from build123d import *

# Parameters (mm, degrees)
BOSS_EXTRUDE1_DEPTH = 6.25
CUT_EXTRUDE1_DEPTH  = 10
BOSS_EXTRUDE2_DEPTH = 6.25
CUT_EXTRUDE2_START  = -1.5
CUT_EXTRUDE2_DEPTH  = 1.5
MOVE_FACE1_BY       = 0.25
SKETCH5_R           = 1.3
CUT_EXTRUDE3_DEPTH  = 0.4
BOSS_EXTRUDE3_DEPTH = 6.25
MOVE_FACE2_BY       = 0.5
MOVE_FACE2_2_BY     = 0.5
CUT_EXTRUDE4_DEPTH  = 13
CUT_EXTRUDE5_START  = -1.5
CUT_EXTRUDE5_DEPTH  = 1.5
BOSS_EXTRUDE4_DEPTH = 6.25
CUT_EXTRUDE6_DEPTH  = 9.000000000000002
FILLET1_R           = 1
FILLET2_R           = 0.3


with BuildPart() as part:
    # Sketch1 → Boss-Extrude1 (new body)
    with BuildSketch(Plane(origin=(0, 0, 0), x_dir=(1, 0, 0), z_dir=(0, 1, 0))):
        with BuildLine():
            Line((-8.500000000000007, 21.49999999999999), (-8.500000000000007, 15.499999999999982))
            Line((-8.500000000000007, 15.499999999999982), (16.645822822062563, 5.999999999999995))
            Line((16.645822822062563, 5.999999999999995), (20.645822822062566, 5.999999999999995))
            ThreePointArc((20.645822822062566, 5.999999999999995), (12.90833064342558, 17.19374886404939), (0, 21.49999999999999))
            Line((0, 21.49999999999999), (-8.500000000000007, 21.49999999999999))
        make_face()
    extrude(amount=BOSS_EXTRUDE1_DEPTH)

    # Sketch2 → Cut-Extrude1 (cut)
    with BuildSketch(Plane(origin=(0, 6.25, 0), x_dir=(1, 0, 0), z_dir=(0, 1, 0))):
        with BuildLine():
            Line((-9.752670250943163, 2.7674418604651105), (-9.752670250943163, 14.499999999999986))
            Line((-9.752670250943163, 14.499999999999986), (8.3e-16, 14.499999999999986))
            ThreePointArc((8.3e-16, 14.499999999999986), (9.22285457500159, 11.188786953390961), (14.233455854041384, 2.7674418604651105))
            Line((14.233455854041384, 2.7674418604651105), (-9.752670250943163, 2.7674418604651105))
        make_face()
    extrude(amount=-CUT_EXTRUDE1_DEPTH, mode=Mode.SUBTRACT)

    # Sketch3 → Boss-Extrude2 (add)
    with BuildSketch(Plane(origin=(0, 6.25, 0), x_dir=(1, 0, 0), z_dir=(0, 1, 0))):
        Polygon((4.469156931645221, 10.801748174518188), (6.3032770804154685, 10.004250036667695), (8.404211615552752, 14.836068669534448), (2.8125557708062745, 17.02319772649103), (0.8009166341047183, 12.396744450219176), (2.6350367828749666, 11.599246312368683), align=None)
    extrude(amount=-BOSS_EXTRUDE2_DEPTH)

    # Sketch4 → Cut-Extrude2 (cut)
    with BuildSketch(Plane.XZ.offset(CUT_EXTRUDE2_START)):
        with BuildLine():
            Line((12.329816757236909, -7.63057132415126), (4.858273185949837, -3.0066464723283906))
            Line((4.858273185949837, -3.0066464723283906), (-2.1755255087838874, -6.757515163827213))
            Line((-2.1755255087838874, -6.757515163827213), (0.39188162426461154, -14.49470347377149))
            ThreePointArc((0.39188162426461154, -14.49470347377149), (7.227688425031692, -12.570223547362334), (12.329816757236909, -7.63057132415126))
        make_face()
    extrude(amount=CUT_EXTRUDE2_DEPTH, mode=Mode.SUBTRACT)

    # Move Face1: a face moved outward by 0.25
    extrude(part.faces().sort_by_distance((3.552096857, 3.875, -11.200497243))[0], amount=MOVE_FACE1_BY, dir=(-0.398749069, 0, 0.917060074))

    # Sketch5 → Cut-Extrude3 (cut)
    with BuildSketch(Plane(origin=(4.560861605165302, 0, -10.489263571615414), x_dir=(0.917060074385124, 0, 0.3987490689252462), z_dir=(-0.3987490689252462, 0, 0.917060074385124))):
        with Locations((-1.20870163918075, 3.2500000000000084)):
            Circle(SKETCH5_R)
    extrude(amount=-CUT_EXTRUDE3_DEPTH, mode=Mode.SUBTRACT)

    # Sketch6 → Boss-Extrude3 (add)
    with BuildSketch(Plane(origin=(0, 6.25, 0), x_dir=(1, 0, 0), z_dir=(0, 1, 0))):
        Polygon((-8.500000000000007, 15.900685410943252), (-8.398385997633637, 15.900685410943252), (-8.398385997633637, 17.900685410943254), (-8.500000000000007, 17.900685410943254), (-10.500000000000009, 17.900685410943254), (-10.500000000000009, 15.900685410943252), align=None)
    extrude(amount=-BOSS_EXTRUDE3_DEPTH)

    # Move Face2: a face moved inward by 0.5
    extrude(part.faces().sort_by_distance((-4.25, 3.125, -21.5))[0], amount=MOVE_FACE2_BY, dir=(0, 0, 1), mode=Mode.SUBTRACT)

    # Move Face2 2: a curved face moved inward by 0.5
    add(Solid.thicken(part.faces().sort_by_distance((12.908330643, 3.125, -17.193748864))[0], -MOVE_FACE2_2_BY), mode=Mode.SUBTRACT)

    # Sketch7 → Cut-Extrude4 (cut)
    with BuildSketch(Plane(origin=(0, 6.25, 0), x_dir=(1, 0, 0), z_dir=(0, 1, 0))):
        with BuildLine():
            Line((-8.500000000000007, 15.900685410943252), (0, 15.900685410943252))
            ThreePointArc((0, 15.900685410943252), (1.1301672935759872, 15.860470309114884), (2.2546178785171396, 15.740028423089157))
            Line((2.2546178785171396, 15.740028423089157), (1.4365096738849472, 13.858508365832973))
            Line((1.4365096738849472, 13.858508365832973), (0.7012293668734065, 12.167479431622894))
            Line((0.7012293668734065, 12.167479431622894), (6.203589813184157, 9.774985018071414))
            Line((6.203589813184157, 9.774985018071414), (7.238188726101288, 12.15439961732261))
            Line((7.238188726101288, 12.15439961732261), (7.94274956604829, 13.774778614149243))
            ThreePointArc((7.94274956604829, 13.774778614149243), (13.653169200208351, 8.150016400490594), (15.89419526397822, 0.45426143168428607))
            Line((15.89419526397822, 0.45426143168428607), (-20.808588691152597, -0.594716444159659))
            Line((-20.808588691152597, -0.594716444159659), (-15.374732718008488, 14.86339738490728))
            Line((-15.374732718008488, 14.86339738490728), (-8.500000000000007, 15.900685410943252))
        make_face()
    extrude(amount=-CUT_EXTRUDE4_DEPTH, mode=Mode.SUBTRACT)

    # Sketch8 → Cut-Extrude5 (cut)
    with BuildSketch(Plane.XZ.offset(CUT_EXTRUDE5_START)):
        with BuildLine():
            Line((14.339308110473954, -6.871392831928589), (1.9043764034639075, -3.0604478341676384))
            Line((1.9043764034639075, -3.0604478341676384), (-4.2629376925202305, -10.324173324993405))
            Line((-4.2629376925202305, -10.324173324993405), (0.7554626751993575, -15.882728754347104))
            ThreePointArc((0.7554626751993575, -15.882728754347104), (8.789998296056245, -13.250197224687337), (14.339308110473954, -6.871392831928589))
        make_face()
    extrude(amount=CUT_EXTRUDE5_DEPTH, mode=Mode.SUBTRACT)

    # Sketch9 → Boss-Extrude4 (add)
    with BuildSketch(Plane(origin=(0, 6.25, 0), x_dir=(1, 0, 0), z_dir=(0, 1, 0))):
        with BuildLine():
            Line((15.70292318448331, 2.500000000000002), (17.725251454235494, 2.500000000000002))
            ThreePointArc((17.725251454235494, 2.500000000000002), (16.78932753436898, 6.209107831207082), (15.086677514257817, 9.634661420966763))
            Line((15.086677514257817, 9.634661420966763), (13.225064123719731, 8.827767297640147))
            ThreePointArc((13.225064123719731, 8.827767297640147), (14.805987713393527, 5.797803408931993), (15.70292318448331, 2.500000000000002))
        make_face()
    extrude(amount=-BOSS_EXTRUDE4_DEPTH)

    # Sketch11 → Cut-Extrude6 (cut)
    with BuildSketch(Plane(origin=(0, 6.25, 0), x_dir=(1, 0, 0), z_dir=(0, 1, 0))):
        with BuildLine():
            Line((7.94274956604829, 13.774778614149243), (11.827692426009557, 10.627205108282226))
            ThreePointArc((11.827692426009557, 10.627205108282226), (10.546532646680365, 13.017226325833846), (7.94274956604829, 13.774778614149243))
        make_face()
        with BuildLine():
            Line((0.7012293668734065, 12.167479431622894), (2.2546178785171413, 15.740028423089157))
            Line((2.2546178785171413, 15.740028423089157), (2.374242599194715, 16.015146445404692))
            ThreePointArc((2.374242599194715, 16.015146445404692), (-0.14915074669056683, 17.00815088772086), (-2.6244470962744906, 15.900685410943252))
            Line((-2.6244470962744906, 15.900685410943252), (0.7012293668734065, 12.167479431622894))
        make_face()
    extrude(amount=-CUT_EXTRUDE6_DEPTH, mode=Mode.SUBTRACT)

    # Fillet1
    fillet1_edges = [part.edges().sort_by_distance(p)[0] for p in [
        (-8.500000000000007, 6.25, -19.45034270547162),
        (18.49489949615255, 0, -5.999999999999995),
        (18.49489949615255, 6.25, -5.999999999999995),
        (-8.500000000000007, 0, -19.45034270547162),
    ]]
    fillet(fillet1_edges, radius=FILLET1_R)

    # Fillet2
    fillet2_edges = [part.edges().sort_by_distance(p)[0] for p in [
        (12.124355652982135, 6.25, -17.146428199482237),
        (-8.500000000000007, 3.1249999999999996, -20.99999999999999),
        (-8.207106781186555, 0.2928932188134522, -20.99999999999999),
        (-8.207106781186555, 5.957106781186548, -20.99999999999999),
        (12.124355652982135, 0, -17.146428199482237),
        (20.124611797498098, 3.125, -5.999999999999995),
        (20.031843616518877, 5.96687308089546, -6.302796311029798),
        (20.03184361651888, 0.2831269191045398, -6.302796311029798),
        (-3.7500000000000036, 0, -20.99999999999999),
        (-3.7500000000000036, 6.25, -20.99999999999999),
    ]]
    fillet(fillet2_edges, radius=FILLET2_R)


solid = part.part
Source: CAD feature listing. Evaluate the final solid. Frame: model axes, mm. A direction names the side the tool comes from. Round coordinates to 2 decimals unless told otherwise and drop trailing zeros. Loops run counter-clockwise (first coordinate to the right, second up) from the corner with the lowest first, then second, coordinate; pieces in that order, holes last. Notation, with made-up numbers: (11, 19) - (32, 19) arc R10 cw to (32, 23) - close; hole circle Ø3 at (29.25, -1). An arc over 180 degrees is marked (long way). Write item = value, one per line. Start each with the question number.
Item 1: Section query B-B on y = 3.75. Output: boundary loops of the cut face in (x, z).
Item 2: First-contact query: pin 1 Ø3 at (y, z) = (2.5, -5.5) entering from -X; pin 2 Ø1 at (y, z) = (1, -9) entering from +X; pin 3 Ø1.8 at (x, z) = (4.5, -12.5) entering from -Y. Flat tips, straight axial feed; report the tip coordinate or a pass-through.
Item 3: Mould query, pull axis Z, two halves, no side actions, for faces 6 (the face through (-7, 3, -15.901)), 7 (the face through (-8.199, 0.285, -19.281)), 8 (the face through (2.58, 2.46, -11.56)), 9 (the face through (-0.11, 3.17, -17.01)). Classes: released by +Z, released by -Z, zero draft, split by the parting line, or undercut.
Item 4: Material intervals for line 1 (Z direction, x = -6.5, y = 5.75); line 2 (Z direction, x = -9, y = 0.75); line 3 (X direction, y = 2.5, z = -16.5), sorted ascending.
Item 5: Reachability of faces 1 (the face through (-8.5, 3, -19)), 2 (the face through (4, 1.5, -13)), 3 (the face through (18, 3, -6)), 4 (the face through (18.119, 5.949, -6.285)), 5 (the face through (18.119, 0.285, -6.301)) from +Z, -Z, +X, -X, +Y, -Y: full face, straight path, thin tool, end or side. Return the list, or none.
Item 6: Section query A-A on x = -5. Output: boundary loops of the cut face in (y, z).
Results list:
q1.outline = (-10.5, -17.9) - (-8.5, -17.9) - (-8.5, -20.7) arc R0.3 ccw to (-8.2, -21) - (0, -21) arc R21 ccw to (20, -6.39) arc R0.3 ccw to (19.72, -6) - (16.87, -6) arc R17.9 ccw to (17.73, -2.5) - (15.7, -2.5) arc R15.9 cw to (11.83, -10.63) arc R3.5 cw to (7.94, -13.77) - (6.2, -9.77) - (4.55, -10.49) - (4.71, -10.86) - (2.51, -11.82) - (2.35, -11.45) - (0.7, -12.17) - (2.37, -16.02) arc R3.5 cw to (-2.62, -15.9) - (-10.5, -15.9) - close
q2.pin_1 = 14.28
q2.pin_2 = 19.2
q2.pin_3 = 1.5
q3.face_6 = released by +Z
q3.face_7 = zero draft
q3.face_8 = undercut
q3.face_9 = undercut
q4.line_1 = -21 to -15.9
q4.line_2 = -17.9 to -15.9
q4.line_3 = -10.5 to -1.89, 1.75 to 12.99
q5.face_1 = -Z, -X, +Y, -Y
q5.face_2 = +Z, -X, -Y
q5.face_3 = +X, +Y, -Y
q5.face_4 = +X, +Y
q5.face_5 = +X, -Y
q6.outline = (0, -20.7) arc R0.3 ccw to (0.3, -21) - (5.95, -21) arc R0.3 ccw to (6.25, -20.7) - (6.25, -15.9) - (0, -15.9) - close
